Check sheet for the drawn part. Datum: minimum x, y, z corner. Units: mm. A direction names the side the tool comes from. Round coordinates to 2 decimals unless told otherwise and drop trailing zeros. Write each loop counter-clockwise with the first axis right and the second up, starting at its lowest first coordinate (ties: lowest second). Pieces come first, ordered by that corner, then holes. Notation, with made-up numbers: M 28,53.5 L 78,53.5 A23 ccw 78,79.5 Z; hole C 22.25,8.5 d8. An arc over 180 degrees is marked long. Put each result on its own line as item: value.
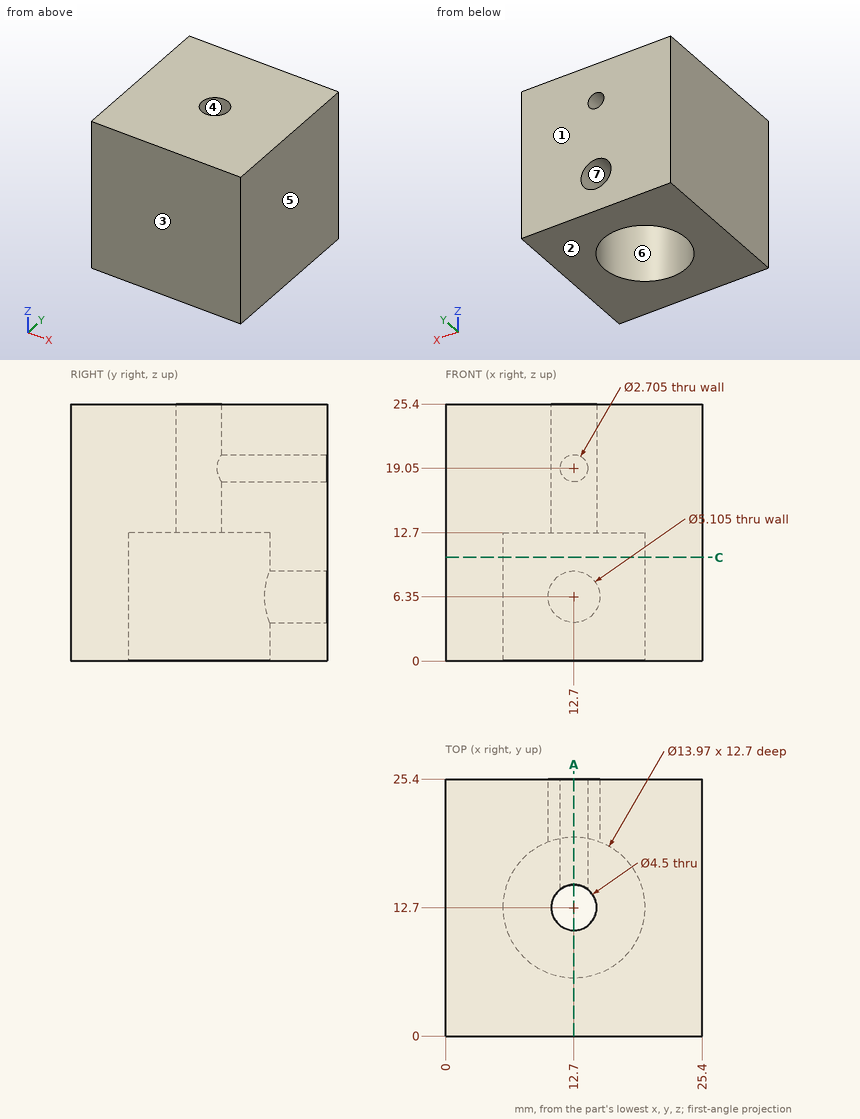
1. Access from +Z, -Z, +X, -X, +Y, -Y to the whole of each face (thin tool, end or side, straight path). Record for the marked faces 5, 6 and 7.
Computed values:
face 5: +Z, -Z, +X, +Y, -Y
face 6: -Z
face 7: +Y
2. Depth check by flat-ended pin: pin 1 Ø3 at (x, z) = (12.7, 6.35) entering from +Y. Enter the tip coordinate at first touch or a pass-through.
Computed values:
pin 1: stops at y = 5.88
3. Release check for a two-part mould opening along Y. For the marked faces 1, 2, 3 and 4 record: +Y half, -Y half, draft (parallel to the pull), parting line (faces both ways), or undercut.
Computed values:
face 1: +Y half
face 2: draft
face 3: -Y half
face 4: undercut
4. Scan lines: probe 1 along Z at (x, y) = (12.7, 22.75); probe 2 along Y at (x, z) = (12.7, 21); probe 3 along Y at (x, z) = (12.7, 5.25) (1 decimal). Record each from-to range of solid material in increasing order.
Computed values:
probe 1: z = 0 to 3.8, 8.9 to 17.7, 20.4 to 25.4
probe 2: y = 0 to 10.45, 14.95 to 25.4
probe 3: y = 0 to 5.7
5. Cross-section at C-C (z = 10.25). Enter the section's corners in (x, y) (1 decimal).
Computed values:
outline: M 0,0 L 25.4,0 L 25.4,25.4 L 0,25.4 Z; hole C 12.7,12.7 d14
6. Cross-section at A-A (x = 12.7). Count the separate pieces of the cut face and the enclosed holes in it, then the cut area to 3 significant figures.
Computed values:
separate pieces: 4
enclosed holes: 0
area: 353 mm2
